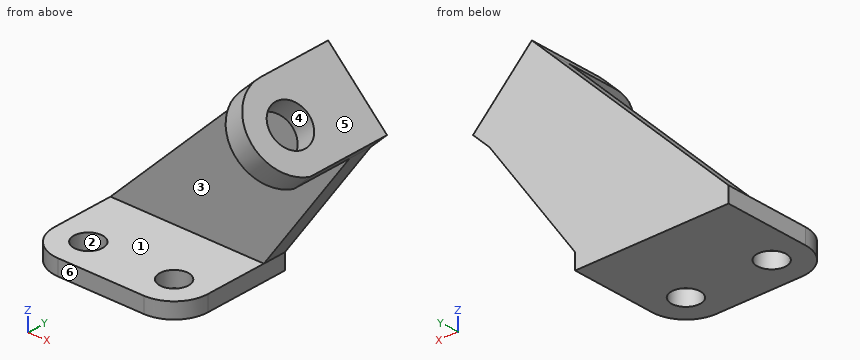
```python
from build123d import *

# Parameters (mm, degrees)
F0_R     = 5.5
F1_DEPTH = 6
F3_DEPTH = 9
F4_R     = 8
F5_DEPTH = 9


with BuildPart() as f1:
    # F0 (on Top) → F1 (new body)
    with BuildSketch(Plane.XY):
        with BuildLine():
            Line((59, 24), (0, 24))
            Line((0, 24), (0, 0))
            ThreePointArc((0, 0), (3.807612, -9.192388), (13, -13))
            Line((13, -13), (46, -13))
            ThreePointArc((46, -13), (55.192388, -9.192388), (59, 0))
            Line((59, 0), (59, 24))
        make_face()
        with Locations((13, 0)):
            Circle(F0_R, mode=Mode.SUBTRACT)
        with Locations((46, 0)):
            Circle(F0_R, mode=Mode.SUBTRACT)
    extrude(amount=F1_DEPTH)

    # F2 (on face) → F3 (join)
    with BuildSketch(Plane(origin=(0, 24, 0), x_dir=(-1, 0, 0), z_dir=(0, 1, 0))):
        Polygon((-91.941125, 52.686292), (-59, 6), (-59, 0), (0, 0), (0, 6), (-69.313708, 75.313708), align=None)
    extrude(amount=F3_DEPTH)

    # F4 (on face) → F5 (join)
    with BuildSketch(Plane(origin=(72.313708, 0, 72.313708), x_dir=(0, 1, 0), z_dir=(0.707107, 0, 0.707107))):
        with BuildLine():
            Line((33, 4.242641), (4, 4.242641))
            ThreePointArc((4, 4.242641), (-12.124515, -9.991795), (0, -27.757359))
            Line((0, -27.757359), (33, -27.757359))
            Line((33, -27.757359), (33, 4.242641))
        make_face()
        with Locations((4, -12.007359)):
            Circle(F4_R, mode=Mode.SUBTRACT)
    extrude(amount=F5_DEPTH)


solid = f1.part
```
Geometry: final body of the model. Coordinates: model frame, mm. Face numbers are marked on the shaded views. A direction names the side the tool comes from. Round coordinates to 2 decimals unless told otherwise and drop trailing zeros. Order: outer loops, then holes, each group sorted by start corner. A loop starts at its lowest first (then second) coordinate and runs counter-clockwise, first axis right, second up. Notation, with made-up numbers: (-8.5, -13.5) - (41.5, -13.5) arc R21 cw to (41.5, 6.5) - close; hole circle Ø11 at (17, -17.75). An arc over 180 degrees is marked (long way). Write item = value, one per line. Start each with the question number.
Q1. Cut plane D-D on y = -9. Return the cut outline in (x, z).
Q2. Access query for the marked faces 1, 2 and 3. Directions: +Z, -Z, +X, -X, +Y, -Y. A direction counts if a zero-diameter tool reaches every point of the face in a straight line with its end or side. Return the directions, or none.
Q3. Cut plane C-C on y = 8.5. Return the cut outline in (x, z), and give its area (3 significant figures).
Q4. Cut plane A-A on y = -1.5. Return the cut outline in (x, z).
Q5. Pull-direction query (Y, two-part tool) for the marked faces 4, 5 and 6; classes: +Y half, -Y half, draft (parallel to the pull), parting line (faces both ways), or undercut.
Q6. Pin query (flat end, axial travel): pin 1 (18.5 mm diameter, centred on x = 16, y = -2, fed in from +Z); pin 2 (4 mm diameter, centred on x = 35.5, z = 16.5, fed in from -Y); pin 3 (1.8 mm diameter, centred on y = 20, z = 1.5, fed in from +X); pin 4 (10 mm diameter, centred on x = 13, y = 0, fed in from +Z). Return the tip coordinate at first contact, or that it passes through.
Q7. Cut plane B-B on x = 11. Return the cut outline in (y, z), and give its area (3 significant figures).
Q8. Ray query, line 1 (Y direction, x = 13, z = 4); line 2 (Y direction, x = 42, z = 19); line 3 (Z direction, x = 45, y = 6). Return the intervals inside material, ascending. Write a range as from..to.
Outcome:
q1.outline = (3.62, 0) - (55.38, 0) - (55.38, 6) - (3.62, 6) - close; (73.91, 70.72) - (87.7, 56.93) - (94.06, 63.29) - (80.27, 77.08) - close
q2.face_1 = +Z, +X, -X, -Y
q2.face_2 = +Z, -Z
q2.face_3 = -X, -Y
q3.outline = (0, 0) - (59, 0) - (59, 6) - (0, 6) - close; (69.31, 75.31) - (76.13, 68.5) - (82.49, 74.86) - (75.68, 81.68) - close; (85.48, 59.15) - (91.94, 52.69) - (98.31, 59.05) - (91.85, 65.51) - close
q3.area = 523 mm^2
q4.outline = (0.09, 0) - (7.71, 0) - (7.71, 6) - (0.09, 6) - close; (18.29, 0) - (40.71, 0) - (40.71, 6) - (18.29, 6) - close; (51.29, 0) - (58.91, 0) - (58.91, 6) - (51.29, 6) - close; (69.99, 74.64) - (76.7, 67.93) - (83.06, 74.3) - (76.36, 81) - close; (84.91, 59.72) - (91.62, 53.01) - (97.98, 59.37) - (91.28, 66.08) - close
q5.face_4 = undercut
q5.face_5 = draft
q5.face_6 = -Y half
q6.pin_1 = 6
q6.pin_2 = 24
q6.pin_3 = 59
q6.pin_4 = through
q7.outline = (-12.85, 0) - (-5.12, 0) - (-5.12, 6) - (-12.85, 6) - close; (5.12, 0) - (33, 0) - (33, 17) - (24, 17) - (24, 6) - (5.12, 6) - close
q7.area = 313 mm^2
q8.line_1 = -13..-5.5, 5.5..33
q8.line_2 = 24..33
q8.line_3 = 0..6
